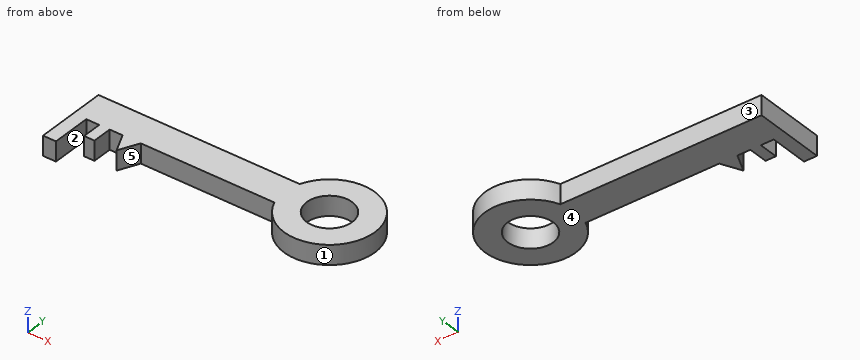
from build123d import *

# Parameters (mm, degrees)
F0_R     = 17.5
F0_W     = 10
F0_H     = 30
F0_W_2   = 8
F0_H_2   = 15
F1_DEPTH = 15


with BuildPart() as f1:
    # F0 (on Top) → F1 (new body)
    with BuildSketch(Plane.XY):
        with BuildLine():
            Line((30.746029, 16.621397), (-124.253971, 16.621397))
            Line((-124.253971, 16.621397), (-124.253971, -8.378603))
            Line((-124.253971, -8.378603), (-114.253971, -8.378603))
            Line((-114.253971, -8.378603), (-104.253971, -8.378603))
            Line((-104.253971, -8.378603), (-96.253971, -8.378603))
            Line((-96.253971, -8.378603), (-86.253971, -8.378603))
            Line((-86.253971, -8.378603), (-72.253971, -8.378603))
            Line((-72.253971, -8.378603), (30.746029, -8.378603))
            ThreePointArc((30.746029, -8.378603), (98.437771, 4.121397), (30.746029, 16.621397))
        make_face()
        with Locations((63.437771, 4.121397)):
            Circle(F0_R, mode=Mode.SUBTRACT)
        with Locations((-119.253971, -23.378603)):
            Rectangle(F0_W, F0_H)
        with Locations((-100.253971, -15.878603)):
            Rectangle(F0_W_2, F0_H_2)
        Polygon((-79.28396, -23.378603), (-72.253971, -8.378603), (-86.253971, -8.378603), align=None)
    extrude(amount=F1_DEPTH)


solid = f1.part
Geometry: final body of the model. Coordinates: model frame, mm. Face numbers are marked on the shaded views. A direction names the side the tool comes from. Give positions to 0.01 mm unless a question says otherwise; leave off trailing zeros. Write each loop counter-clockwise with the first axis right and the second up, starting at its lowest first coordinate (ties: lowest second). Pieces come first, ordered by that corner, then holes.
(1) Cut plane C-C, the plane z = 10.75. Return loops of the section in (x, y), then the cut area to 3 significant figures.
(2) Mould query, pull axis X, two halves, no side actions, for the marked faces 4 and 5. Classes: released by +X, released by -X, zero draft, split by the parting line, or undercut.
(3) Access query for the marked faces 1, 2 and 3. Directions: +Z, -Z, +X, -X, +Y, -Y. A direction counts if a zero-diameter tool reaches every point of the face in a straight line with its end or side. Return the directions, or none.
(4) Cut plane D-D, the plane y = -33. Return loops of the section in (x, z), then the cut area to 3 significant figures.
(5) First-contact query: P1, Ø4, axis at x = -59, z = 11.5, coming from the +Y side; P2, Ø4, axis at y = 21.5, z = 8, coming from the -X side; P3, Ø8, axis at x = -110, z = 9, coming from the -Y side. Flat tips, straight axial feed; report the tip coordinate or a pass-through.
(6) Cut plane B-B, the plane x = 53. Return loops of the section in (y, z), then the cut area to 3 significant figures.
(7) Ray query, line 1 (X direction, y = 3.5, z = 9.25); line 2 (Y direction, x = -50, z = 11.5); line 3 (X direction, y = 17, z = 3.25). Return the intervals inside material, ascending.
(8) Cut plane A-A, the plane y = 10.5. Return loops of the section in (x, z), then the cut area to 3 significant figures.
Values follow:
1. outline: (-124.25, -38.38) - (-114.25, -38.38) - (-114.25, -8.38) - (-104.25, -8.38) - (-104.25, -23.38) - (-96.25, -23.38) - (-96.25, -8.38) - (-86.25, -8.38) - (-79.28, -23.38) - (-72.25, -8.38) - (30.75, -8.38) arc R35 ccw (long way) to (30.75, 16.62) - (-124.25, 16.62) - close; hole circle Ø35 at (63.44, 4.12)
1. area: 7,250 mm2
2. face 4: zero draft
2. face 5: undercut
3. face 1: +Z, -Z
3. face 2: +Z, -Z, -Y
3. face 3: +Z, -Z, -X, +Y
4. outline: (-124.25, 0) - (-114.25, 0) - (-114.25, 15) - (-124.25, 15) - close
4. area: 150 mm2
5. P1: stops at y = 16.62
5. P2: stops at x = 32
5. P3: stops at y = -8.38
6. outline: (-29.29, 0) - (-9.93, 0) - (-9.93, 15) - (-29.29, 15) - close; (18.17, 0) - (37.53, 0) - (37.53, 15) - (18.17, 15) - close
6. area: 581 mm2
7. line 1: x = -124.25 to 45.95, 80.93 to 98.43
7. line 2: y = -8.38 to 16.62
7. line 3: x = 30.89 to 51.59, 75.29 to 95.98
8. outline: (-124.25, 0) - (47.14, 0) - (47.14, 15) - (-124.25, 15) - close; (79.73, 0) - (97.85, 0) - (97.85, 15) - (79.73, 15) - close
8. area: 2,840 mm2
